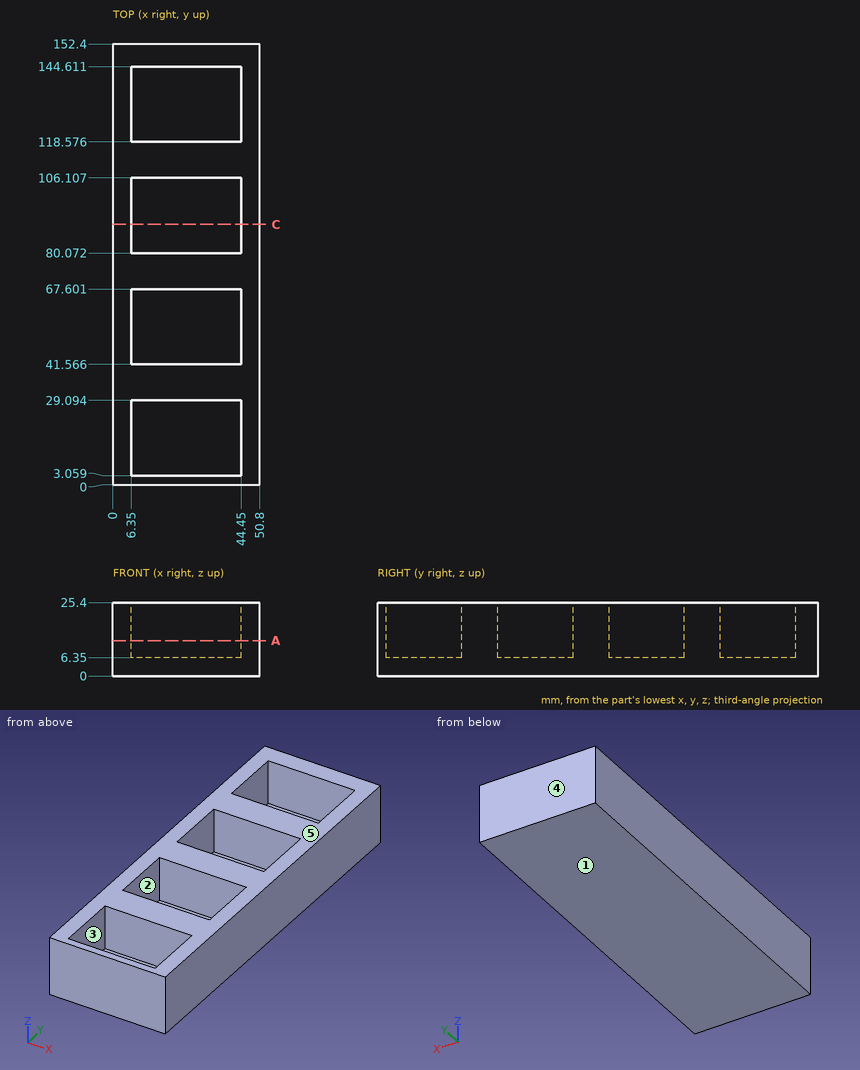
Input: dimensioned drawing with shaded views. Units: mm. Origin: part minimum x, y, z. A direction names the side the tool comes from. Give positions to 0.01 mm unless a question says otherwise; leave off trailing zeros. Loops run counter-clockwise (first coordinate to the right, second up) from the corner with the lowest first, then second, coordinate; pieces in that order, holes last. Notation, with made-up numbers: (-26.5, 70) -> (15.5, 70) arc R17 ccw to (15.5, 80) -> close; hole circle Ø5 at (40, 55). An arc over 180 degrees is marked (long way). Use a Markdown table: item, result. Add a question column.
1) Reachability of the marked faces 1 and 2 from +Z, -Z, +X, -X, +Y, -Y: full face, straight path, thin tool, end or side. Return the list, or none.
2) Section query A-A, the plane z = 12.25. Count the separate pieces of the cut face and the enclosed holes in it, then the cut area to 3 significant figures.
3) Section query C-C, the plane y = 90. Return the cut outline in (x, z).
4) Pull-direction query (Y, two-part tool) for the marked faces 3, 4 and 5; classes: +Y half, -Y half, draft (parallel to the pull), parting line (faces both ways), or undercut.
5) First-contact query: pin 1 (21 mm diameter, centred on x = 33.5, y = 61, fed in from +Z); pin 2 (2 mm diameter, centred on x = 29, y = 82, fed in from +Z). Flat tips, straight axial feed; report the tip coordinate or a pass-through.
6) Line query: line 1 along Y through (x, z) = (22.5, 16.75) (1 decimal); line 2 along X through (y, z) = (58.5, 11); line 3 along Z through (x, y) = (17, 17). Output: solid intervals per line, ascending. Write a range as [from, to].
Numbers:
| question | item | result |
|---|---|---|
| 1 | face 1 | -Z, +X, -X, +Y, -Y |
| 1 | face 2 | +Z |
| 2 | separate pieces | 1 |
| 2 | enclosed holes | 4 |
| 2 | area | 3,770 mm2 |
| 3 | outline | (0, 0) -> (50.8, 0) -> (50.8, 25.4) -> (44.45, 25.4) -> (44.45, 6.35) -> (6.35, 6.35) -> (6.35, 25.4) -> (0, 25.4) -> close |
| 4 | face 3 | undercut |
| 4 | face 4 | +Y half |
| 4 | face 5 | draft |
| 5 | pin 1 | stops at z = 25.4 |
| 5 | pin 2 | stops at z = 6.35 |
| 6 | line 1 | y = [0, 3.1], [29.1, 41.6], [67.6, 80.1], [106.1, 118.6], [144.6, 152.4] |
| 6 | line 2 | x = [0, 6.35], [44.45, 50.8] |
| 6 | line 3 | z = [0, 6.35] |
